Verification items for the finished model (mm, model axes). A direction names the side the tool comes from. Give positions to 0.01 mm unless a question says otherwise; leave off trailing zeros. Order: outer loops, then holes, each group sorted by start corner. A loop starts at its lowest first (then second) coordinate and runs counter-clockwise, first axis right, second up. Notation, with made-up numbers: M 29,39.25 L 88,39.25 A17 ccw 88,43.25 Z; hole C 19.25,-35.75 d8. An arc over 180 degrees is marked long. Answer as a JSON object with one key per item and string values.
```python
from build123d import *

# Parameters (mm, degrees)
BOSS_EXTRUDE1_DEPTH = 4
SKETCH2_R           = 2
CUT_EXTRUDE1_DEPTH  = 24.366642891
FILLET1_RADIUS      = 4
FILLET1_LENGTH      = 4
FILLET2_RADIUS      = 4
FILLET2_LENGTH      = 4
CUT_EXTRUDE2_START  = 3.8
SKETCH3_R           = 3.6
CUT_EXTRUDE2_DEPTH  = 20.566642908


with BuildPart() as part:
    # Sketch1 → Boss-Extrude1 (new, symmetric)
    with BuildSketch(Plane.XY):
        with BuildLine():
            Line((-19, 0), (-9, 0))
            ThreePointArc((-9, 0), (0, 9), (9, 0))
            Line((9, 0), (19, 0))
            Line((19, 0), (19, 4))
            Line((19, 4), (14.071247279, 4))
            ThreePointArc((14.071247279, 4), (12.724207514, 4.393941152), (11.801691267, 5.451612903))
            ThreePointArc((11.801691267, 5.451612903), (0, 13), (-11.801691267, 5.451612903))
            ThreePointArc((-11.801691267, 5.451612903), (-12.724207514, 4.393941152), (-14.071247279, 4))
            Line((-14.071247279, 4), (-19, 4))
            Line((-19, 4), (-19, 0))
        make_face()
    extrude(amount=BOSS_EXTRUDE1_DEPTH, both=True)

    # Sketch2 → Cut-Extrude1 (cut, through all)
    with BuildSketch(Plane(origin=(0, 0, 0), x_dir=(1, 0, 0), z_dir=(0, 1, 0))):
        with Locations(Location((15, 0, 0), (0, 0, 117.669868627))):
            Circle(SKETCH2_R)
        with Locations(Location((-15, 0, 0), (0, 0, 62.330131378))):
            Circle(SKETCH2_R)
    extrude(amount=CUT_EXTRUDE1_DEPTH, mode=Mode.SUBTRACT)

    # Fillet1: full round fillet: the end face becomes a half cylinder, R = half its width
    fillet1_face = Plane((19, 2, 0), x_dir=(0, 1, 0), z_dir=(1, 0, 0))  # on the end face: x along it, z out of the body
    fillet1_slab = fillet1_face.offset(-FILLET1_RADIUS / 2) * Box(FILLET1_LENGTH, 2 * FILLET1_RADIUS, FILLET1_RADIUS, mode=Mode.PRIVATE)  # the body's end, R deep
    fillet1_round = Plane((15, 2, 0), x_dir=(1, 0, 0), z_dir=(0, 1, 0)) * Cylinder(FILLET1_RADIUS, FILLET1_LENGTH, mode=Mode.PRIVATE)  # its axis R under the face
    add(fillet1_slab - fillet1_round, mode=Mode.SUBTRACT)

    # Fillet2: full round fillet: the end face becomes a half cylinder, R = half its width
    fillet2_face = Plane((-19, 2, 0), x_dir=(0, -1, 0), z_dir=(-1, 0, 0))  # on the end face: x along it, z out of the body
    fillet2_slab = fillet2_face.offset(-FILLET2_RADIUS / 2) * Box(FILLET2_LENGTH, 2 * FILLET2_RADIUS, FILLET2_RADIUS, mode=Mode.PRIVATE)  # the body's end, R deep
    fillet2_round = Plane((-15, 2, 0), x_dir=(-1, 0, 0), z_dir=(0, -1, 0)) * Cylinder(FILLET2_RADIUS, FILLET2_LENGTH, mode=Mode.PRIVATE)  # its axis R under the face
    add(fillet2_slab - fillet2_round, mode=Mode.SUBTRACT)

    # Sketch3 → Cut-Extrude2 (cut, through all)
    with BuildSketch(Plane(origin=(0, 0, 0), x_dir=(1, 0, 0), z_dir=(0, 1, 0)).offset(CUT_EXTRUDE2_START)):
        with Locations(Location((-15, 0, 0), (0, 0, 75.049356593))):
            Circle(SKETCH3_R)
        with Locations(Location((15, 0, 0), (0, 0, 104.950643407))):
            Circle(SKETCH3_R)
    extrude(amount=CUT_EXTRUDE2_DEPTH, mode=Mode.SUBTRACT)


solid = part.part
```
Q1. Release check for a two-part mould opening along Z. For faces 4 (the face through (-0.2, 9.5, 4)), 5 (the face through (16.93, 1.87, -0.52)), 6 (the face through (-0.2, 9.5, -4)), 7 (the face through (12.8, 0, 0.1)) record: +Z half, -Z half, draft (parallel to the pull), parting line (faces both ways), or undercut.
Resolved:
{"face 4": "+Z half", "face 5": "undercut", "face 6": "-Z half", "face 7": "draft"}
Q2. Tool access check on faces 1 (the face through (-18.71, 4, -0.57)), 2 (the face through (-11.4, 4.6, -0.1)), 3 (the face through (18.74, 4, 0.31)). Record the directions out of +Z, -Z, +X, -X, +Y, -Y that give a thin tool (end or side, any length) a straight path to the whole face; none if there is none.
Resolved:
{"face 1": "+Z, -Z, -X, +Y", "face 2": "+Y", "face 3": "+Z, -Z, +X, +Y"}
Q3. Section check D-D on z = 2.75. Record the cut outline in (x, y), then the cut area to 3 significant figures.
Resolved:
{"outline": "M -17.9,0 L -9,0 A9 cw 9,0 L 17.9,0 L 17.9,4 L 17.32,4 L 17.32,3.8 L 12.68,3.8 L 12.68,4.43 A2.5 cw 11.8,5.45 A13 ccw -11.8,5.45 A2.5 cw -12.68,4.43 L -12.68,3.8 L -17.32,3.8 L -17.32,4 L -17.9,4 Z", "area": "178 mm²"}
Q4. Gauge pin test, flat ends, axial feed: pin 1 Ø2.5 at (x, z) = (16, 0.5) entering from +Y; pin 2 Ø4 at (x, z) = (2.5, 2) entering from +Y; pin 3 Ø2.5 at (x, z) = (-17.5, 0) entering from +Y; pin 4 Ø2 at (y, z) = (4.5, 0.5) entering from -X. Record the tip position at first contact, or that the pin passes through.
Resolved:
{"pin 1": "stops at y = 3.8", "pin 2": "stops at y = 12.99", "pin 3": "stops at y = 4", "pin 4": "stops at x = -19"}
Q5. Material ranges on L1, parallel to X at y = 1.75, z = -1.5; L2, parallel to X at y = 2.25, z = 0; L3, parallel to Z at x = -15, y = 0.95, recorded low to high.
Resolved:
{"L1": "x = -18.71 to -16.32, -13.68 to -8.83, 8.83 to 13.68, 16.32 to 18.71", "L2": "x = -19 to -17, -13 to -8.71, 8.71 to 13, 17 to 19", "L3": "z = -4 to -2, 2 to 4"}
Q6. Section check A-A on z = 0. Record the cut outline in (x, y).
Resolved:
{"outline": "M -19,0 L -17,0 L -17,3.8 L -18.6,3.8 L -18.6,4 L -19,4 Z; M -13,0 L -9,0 A9 cw 9,0 L 13,0 L 13,3.8 L 11.4,3.8 L 11.4,6.25 A13 ccw -11.4,6.25 L -11.4,3.8 L -13,3.8 Z; M 17,0 L 19,0 L 19,4 L 18.6,4 L 18.6,3.8 L 17,3.8 Z"}
Q7. Section check B-B on y = 5. Record the cut outline in (x, z).
Resolved:
{"outline": "M -12.07,-4 L -7.48,-4 L -7.48,4 L -12.07,4 L -12.07,2.09 A3.6 cw -12.07,-2.09 Z; M 7.48,-4 L 12.07,-4 L 12.07,-2.09 A3.6 cw 12.07,2.09 L 12.07,4 L 7.48,4 Z"}
Q8. Section check C-C on x = 15.5. Record the cut outline in (y, z), then the cut area to 3 significant figures.
Resolved:
{"outline": "M 0,-3.97 L 4,-3.97 L 4,-3.57 L 3.8,-3.57 L 3.8,-1.94 L 0,-1.94 Z; M 0,1.94 L 3.8,1.94 L 3.8,3.57 L 4,3.57 L 4,3.97 L 0,3.97 Z", "area": "15.6 mm²"}
